Design review of the part shown in the three views and the two pictorial views. Dimensions are in mm from the part's minimum x, y and z. A direction names the side the tool comes from. Coordinates: 2 decimals unless noted, no trailing zeros. Loops run counter-clockwise (first coordinate to the right, second up) from the corner with the lowest first, then second, coordinate; pieces in that order, holes last. Notation, with made-up numbers: M 6.5,69.5 L 37.5,69.5 A18 cw 37.5,96.5 Z; hole C 20,40.25 d3. An arc over 180 degrees is marked long. Write item = value, one per line. Start each with the question number.
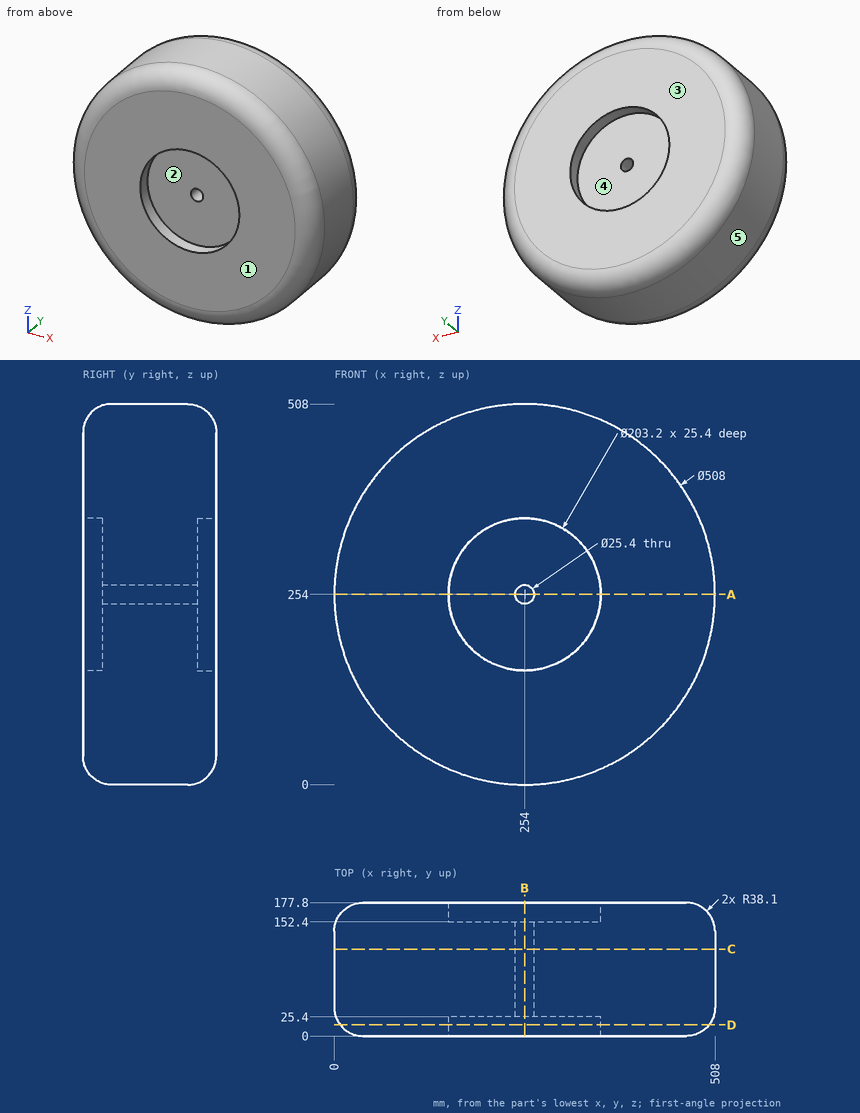
(1) Take a section at B-B (x = 254). State the section outline as (y, z) points, plus the area to 3 significant figures.
(2) Insertion check: pin 1 (4 mm diameter, centred on x = 390, y = 153.5, fed in from +Z); pin 2 (1 mm diameter, centred on y = 134.5, z = 348.5, fed in from +X); pin 3 (6 mm diameter, centred on x = 169.5, z = 354.5, fed in from -Y); pin 4 (8 mm diameter, centred on x = 180, z = 215, fed in from -Y). Each pin has a flat end and moves straight along its axis. Give the tip position at first contact, or say it passes through.
(3) To check wall thickness, follow L1, parallel to Z at x = 254, y = 113; L2, parallel to Z at x = 254, y = 5; L3, parallel to Y at x = 326, z = 189.5. State the ranges of each line that lie inside material, in increasing order.
(4) Tool access review of the marked faces 1 and 2: name each direction out of +Z, -Z, +X, -X, +Y, -Y from which nothing blocks a thin tool from reaching the whole face with its end or side.
(5) Mouldability with a two-part tool opening along X and no side actions: class the marked faces 3, 4 and 5 as +X half, -X half, draft (parallel to the pull), parting line (faces both ways), or undercut.
(6) Take a section at D-D (y = 15). State the section outline as (x, z) points.
(7) Take a section at C-C (y = 116). State the section outline as (x, z) points.
(8) Take a section at A-A (z = 254). State the section outline as (x, y) points, plus the area to 3 significant figures.
Results list:
q1.outline = M 0,38.1 A38.1 ccw 38.1,0 L 139.7,0 A38.1 ccw 177.8,38.1 L 177.8,152.4 L 152.4,152.4 L 152.4,241.3 L 25.4,241.3 L 25.4,152.4 L 0,152.4 Z; M 0,355.6 L 25.4,355.6 L 25.4,266.7 L 152.4,266.7 L 152.4,355.6 L 177.8,355.6 L 177.8,469.9 A38.1 ccw 139.7,508 L 38.1,508 A38.1 ccw 0,469.9 Z
q1.area = 75,500 mm^2
q2.pin_1 = 467
q2.pin_2 = 489.97
q2.pin_3 = 0
q2.pin_4 = 25.4
q3.L1 = 0 to 241.3, 266.7 to 508
q3.L2 = 19.23 to 152.4, 355.6 to 488.77
q3.L3 = 25.4 to 152.4
q4.face_1 = +Z, -Z, +X, -X, -Y
q4.face_2 = -Y
q5.face_3 = draft
q5.face_4 = undercut
q5.face_5 = parting line
q6.outline = C 254,254 d492.4; hole C 254,254 d203.2
q7.outline = C 254,254 d508; hole C 254,254 d25.4
q8.outline = M 0,38.1 A38.1 ccw 38.1,0 L 152.4,0 L 152.4,25.4 L 241.3,25.4 L 241.3,152.4 L 152.4,152.4 L 152.4,177.8 L 38.1,177.8 A38.1 ccw 0,139.7 Z; M 266.7,25.4 L 355.6,25.4 L 355.6,0 L 469.9,0 A38.1 ccw 508,38.1 L 508,139.7 A38.1 ccw 469.9,177.8 L 355.6,177.8 L 355.6,152.4 L 266.7,152.4 Z
q8.area = 75,500 mm^2
